Design review of the part shown in the three views and the two pictorial views. Dimensions are in mm from the part's minimum x, y and z. A direction names the side the tool comes from. Give positions to 0.01 mm unless a question says otherwise; leave off trailing zeros. Loops run counter-clockwise (first coordinate to the right, second up) from the corner with the lowest first, then second, coordinate; pieces in that order, holes last. Notation, with made-up numbers: (18.5, 80) -> (42.5, 80) arc R24 ccw to (42.5, 116) -> close; hole circle Ø10 at (29.5, 19.25). An arc over 180 degrees is marked (long way). Answer as CSV lines item,"result".
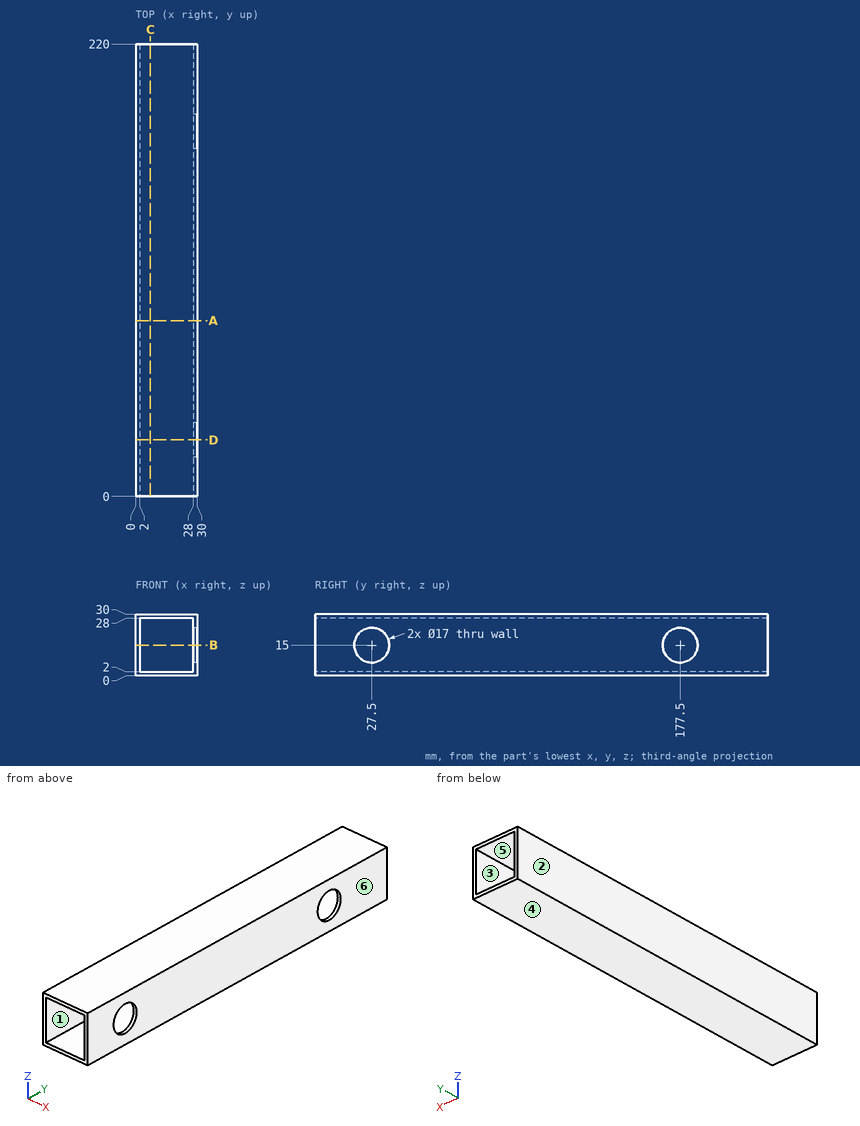
Q1. We need section B-B, the plane z = 15. State the section outline as (x, y) points, and give its area (3 significant figures).
Filled sheet:
outline,"(0, 0) -> (2, 0) -> (2, 220) -> (0, 220) -> close; (28, 0) -> (30, 0) -> (30, 19) -> (28, 19) -> close; (28, 36) -> (30, 36) -> (30, 169) -> (28, 169) -> close; (28, 186) -> (30, 186) -> (30, 220) -> (28, 220) -> close"
area,"812 mm^2"
Q2. For the marked faces 5 and 6, list the 3-axis set-ups (+Z, -Z, +X, -X, +Y, -Y) from which the entire face can be reached by the end or side of a thin tool; tool diameter is ignored.
Filled sheet:
face 5,"+Y, -Y"
face 6,"+Z, -Z, +X, +Y, -Y"
Q3. The part is to be moulded in two halves that separate along X. For the marked faces 1, 2, 3 and 4, say which applies: pulls with the +X half, pulls with the -X half, needs draft (parallel to the pull), parting line crosses it, or undercut.
Filled sheet:
face 1,"undercut"
face 2,"pulls with the -X half"
face 3,"undercut"
face 4,"needs draft"
Q4. To check wall thickness, follow probe 1 along Y at (x, z) = (29.2, 15); probe 2 along Z at (x, y) = (14.5, 176); probe 3 along Z at (x, y) = (29.05, 27.5). State the ranges of each line that lie inside material, in increasing order. Write a range as from..to.
Filled sheet:
probe 1,"y = 0..19, 36..169, 186..220"
probe 2,"z = 0..2, 28..30"
probe 3,"z = 0..6.5, 23.5..30"
Q5. We need section D-D, the plane y = 27.5. State the section outline as (x, z) points.
Filled sheet:
outline,"(0, 0) -> (30, 0) -> (30, 6.5) -> (28, 6.5) -> (28, 2) -> (2, 2) -> (2, 28) -> (28, 28) -> (28, 23.5) -> (30, 23.5) -> (30, 30) -> (0, 30) -> close"
Q6. Clearance check with a flat-ended pin moving along its axis: pin 1 Ø1 at (x, y) = (15, 117) entering from -Z. State where the tip first meets the part, or that it passes through.
Filled sheet:
pin 1,"stops at z = 0"
Q7. We need section C-C, the plane x = 7.25. State the section outline as (y, z) points.
Filled sheet:
outline,"(0, 0) -> (220, 0) -> (220, 2) -> (0, 2) -> close; (0, 28) -> (220, 28) -> (220, 30) -> (0, 30) -> close"
Q8. We need section A-A, the plane y = 85.5. State the section outline as (x, z) points, and give its area (3 significant figures).
Filled sheet:
outline,"(0, 0) -> (30, 0) -> (30, 30) -> (0, 30) -> close; hole (2, 2) -> (28, 2) -> (28, 28) -> (2, 28) -> close"
area,"224 mm^2"
